Autodesk Inventor part; units mm, degrees
ref_plane "XY Plane" through (0, 0, 0) normal (0, 0, 1) x (1, 0, 0)
sketch "Sketch1" plane through (0, 0, 0) normal (1, 0, 0) x (0, 1, 0)
  line L0 (-25.4, -25.4) -> (-25.4, 25.4)
  line L1 (-25.4, 25.4) -> (25.4, 25.4)
  line L2 (25.4, 25.4) -> (25.4, -25.4)
  line L3 (25.4, -25.4) -> (-25.4, -25.4)
  line L4 (-25.4, -25.4) -> (25.4, 25.4) construction
  line L5 (-25.4, 25.4) -> (25.4, -25.4) construction
  point P0 (0, 0)
  dimension "d0" = 50.8
  dimension "d1" = 50.8
extrude "Extrusion1" add sketch "Sketch1" along normal mid plane 50.8
sketch "Sketch2" plane through (-25.4, -25.4, 25.4) normal (0, 0, 1) x (1, 0, 0)
  circle A0 centre (25.4, 25.4) radius 5.2705
  dimension "d4" = 10.541
extrude "Extrusion2" cut sketch "Sketch2" against normal through all
properties part number "cylinderForCopy"
Could you check a few things on this model? Use its own coordinates, in mm. Round coordinates to 2 decimals unless told otherwise and drop trailing zeros. Write each loop counter-clockwise with the first axis right and the second up, starting at its lowest first coordinate (ties: lowest second). Pieces come first, ordered by that corner, then holes. Notation, with made-up numbers: M 72.25,7.5 L 130.25,7.5 A15 ccw 130.25,18.5 Z; hole C -24.5,14 d7. An arc over 180 degrees is marked long. Answer in a Markdown table with one row per item. Add a question column.
Q1. If we mould it in two halves opening along Y, with no side actions, what happens to faces 1 (the cylindrical face through (5.03, 1.58, 0.36)), 2 (the flat face through (25.4, 0, 0)), 3 (the flat face through (0, 25.4, 0))? For each: +Y half, -Y half, draft (parallel to the pull), parting line (faces both ways), or undercut.
Q2. Imagine slicing it at C-C (z = 5). Please give me the cut outline in (x, y).
Q3. If I drill on line 1 (Y direction, x = 0, z = 5); line 2 (X direction, y = 3.5, z = -9.5); line 3 (Y direction, x = -2.5, z = 23.5), over which ranges is the centre line in solid material (lowest first)? Write a range as from..to.
Q4. Imagine slicing it at A-A (y = 0). Please give me the cut outline in (x, z).
Values:
| question | item | result |
|---|---|---|
| 1 | face 1 | undercut |
| 1 | face 2 | draft |
| 1 | face 3 | +Y half |
| 2 | outline | M -25.4,-25.4 L 25.4,-25.4 L 25.4,25.4 L -25.4,25.4 Z; hole C 0,0 d10.54 |
| 3 | line 1 | -25.4..-5.27, 5.27..25.4 |
| 3 | line 2 | -25.4..-3.94, 3.94..25.4 |
| 3 | line 3 | -25.4..-4.64, 4.64..25.4 |
| 4 | outline | M -25.4,-25.4 L -5.27,-25.4 L -5.27,25.4 L -25.4,25.4 Z; M 5.27,-25.4 L 25.4,-25.4 L 25.4,25.4 L 5.27,25.4 Z |
